The model under review builds one solid part; all positions refer to its coordinate system, in mm. Face numbers are marked on the shaded views. A direction names the side the tool comes from. Round coordinates to 2 decimals unless told otherwise and drop trailing zeros. Order: outer loops, then holes, each group sorted by start corner. A loop starts at its lowest first (then second) coordinate and runs counter-clockwise, first axis right, second up. Notation, with made-up numbers: (-6.5, 29.25) -> (34.5, 29.25) arc R25 cw to (34.5, 61.25) -> close; hole circle Ø7 at (52.5, -33). An arc over 180 degrees is marked (long way). Return JSON: item names as keys, results as strings. Group by question number.
from build123d import *

# Parameters (mm, degrees)
F0_R          = 9.75
F1_DEPTH      = 25.4
F2_R          = 8.255
F3_DEPTH      = 25.4
F4_R          = 15.875
F4_R_2        = 9.75
F5_DEPTH      = 2.54
F6_R          = 15.875
F6_R_2        = 12
F7_DEPTH      = 9.525
F9_DEPTH      = 25.4
F9_DEPTH_BACK = 25.4


with BuildPart() as f1:
    # F0 (on Top) → F1 (new body)
    with BuildSketch(Plane.XY):
        Circle(F0_R)
    extrude(amount=F1_DEPTH)

    # F2 (on face) → F3 (cut)
    with BuildSketch(Plane.XY.offset(25.4)):
        Circle(F2_R)
    extrude(amount=-F3_DEPTH, mode=Mode.SUBTRACT)

    # F4 (on face) → F5 (join)
    with BuildSketch(Plane(origin=(0, 0, 0), x_dir=(1, 0, 0), z_dir=(0, 0, -1))):
        Circle(F4_R)
        Circle(F4_R_2, mode=Mode.SUBTRACT)
    extrude(amount=-F5_DEPTH)

    # F6 (on face) → F7 (join)
    with BuildSketch(Plane.XY.offset(2.54)):
        Circle(F6_R)
        Circle(F6_R_2, mode=Mode.SUBTRACT)
    extrude(amount=F7_DEPTH)

    # F8 (on Right) → F9 (cut, two sides)
    with BuildSketch(Plane.YZ) as f9_sk:
        with BuildLine():
            ThreePointArc((0, 5.3025), (1.4142135624, 5.8882864376), (2, 7.3025))
            ThreePointArc((2, 7.3025), (-1.4142135624, 8.7167135624), (0, 5.3025))
        make_face()
    extrude(amount=-F9_DEPTH, mode=Mode.SUBTRACT)
    extrude(f9_sk.sketch, amount=F9_DEPTH_BACK, mode=Mode.SUBTRACT)


solid = f1.part
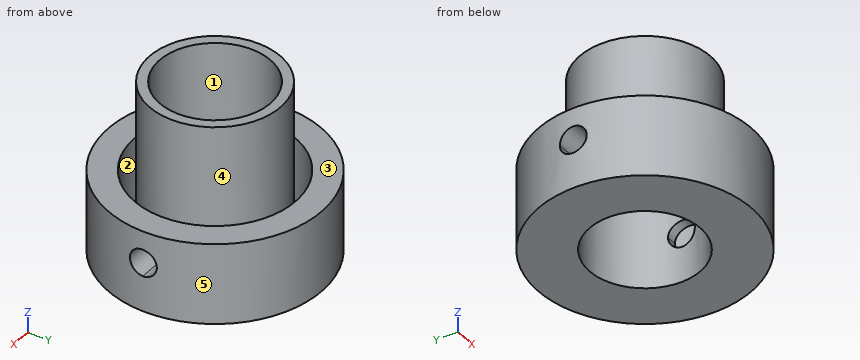
Item 1: Wall thickness on line 1 along X through (y, z) = (0, 10) (3 decimals); line 2 along Z through (x, y) = (8.8, 0); line 3 along Z through (x, y) = (12.95, 0) (1 decimal): over which ranges is each line inside the solid? List them lowest first.
Item 2: Insertion check: pin 1 Ø4.5 at (y, z) = (0, 7.3) entering from -X (3 decimals); pin 2 Ø1 at (x, z) = (-6, 17.5) entering from -Y; pin 3 Ø10 at (x, z) = (-11, 10) entering from -Y; pin 4 Ø3 at (y, z) = (-7, 15.5) entering from +X. Each pin has a flat end and moves straight along its axis. Give the tip position at first contact, or say it passes through.
Item 3: Consider section B-B on z = 4.5. State the section outline as (x, y) points (3 decimals).
Item 4: Consider section A-A on x = 0. State the section outline as (y, z) points (3 decimals), plus the area to 3 significant figures.
Item 5: Consider section D-D on z = 15.25. State the section outline as (x, y) points (3 decimals), plus the area to 3 significant figures.
Item 6: For the marked faces 1 and 2, list the 3-axis set-ups (+Z, -Z, +X, -X, +Y, -Y) from which the entire face can be reached by the end or side of a thin tool; tool diameter is ignored.
Item 7: The part is to be moulded in two halves that separate along X. For the marked faces 3, 4 and 5, say which applies: +X half, -X half, draft (parallel to the pull), parting line (faces both ways), or undercut.
Item 8: Consider section C-C on x = -11. State the section outline as (y, z) points (3 decimals).
Values:
{
 "1": {"line 1": "-15.875 to -12, -9.75 to -8.255, 8.255 to 9.75, 12 to 15.875", "line 2": "0 to 5.3, 9.3 to 25.4", "line 3": "0 to 5.3, 9.3 to 12.1"},
 "2": {"pin 1": "x = -15.875", "pin 2": "y = -8.05", "pin 3": "y = -14.7", "pin 4": "x = 8.05"},
 "3": {"outline": "circle Ø31.75 at (0, 0); circle Ø19.5 at (0, 0); hole circle Ø24 at (0, 0); hole circle Ø16.51 at (0, 0)"},
 "4": {"outline": "(-15.875, 0) -> (-8.255, 0) -> (-8.255, 25.4) -> (-9.75, 25.4) -> (-9.75, 2.54) -> (-12, 2.54) -> (-12, 12.065) -> (-15.875, 12.065) -> close; (8.255, 0) -> (15.875, 0) -> (15.875, 12.065) -> (12, 12.065) -> (12, 2.54) -> (9.75, 2.54) -> (9.75, 25.4) -> (8.255, 25.4) -> close", "area": "181 mm^2"},
 "5": {"outline": "circle Ø19.5 at (0, 0); hole circle Ø16.51 at (0, 0)", "area": "84.6 mm^2"},
 "6": {"face 1": "+Z, -Z", "face 2": "+Z"},
 "7": {"face 3": "draft", "face 4": "undercut", "face 5": "parting line"},
 "8": {"outline": "(-11.446, 0) -> (11.446, 0) -> (11.446, 12.065) -> (4.796, 12.065) -> (4.796, 2.54) -> (-4.796, 2.54) -> (-4.796, 12.065) -> (-11.446, 12.065) -> close"}
}
